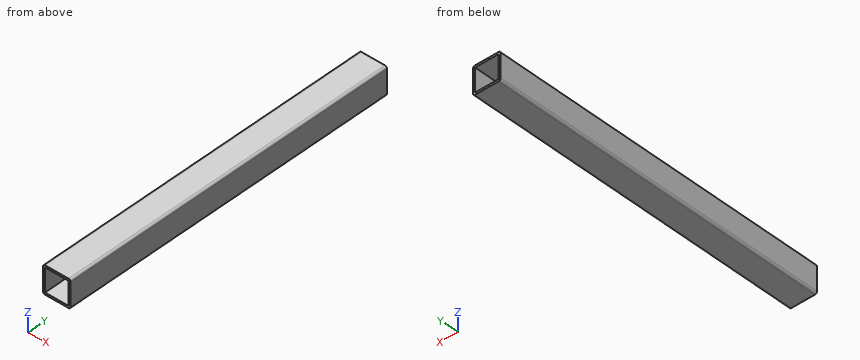
```python
from build123d import *

# Parameters (mm, degrees)
F0_W     = 34
F0_H     = 34
F1_DEPTH = 500


with BuildPart() as f1:
    # F0 (on Front) → F1 (new body)
    with BuildSketch(Plane.XZ):
        with BuildLine():
            ThreePointArc((19.779984, 17.078975), (18.901304, 19.200296), (16.779984, 20.078975))
            Line((16.779984, 20.078975), (-17.220016, 20.078975))
            ThreePointArc((-17.220016, 20.078975), (-19.341336, 19.200296), (-20.220016, 17.078975))
            Line((-20.220016, 17.078975), (-20.220016, -16.921025))
            ThreePointArc((-20.220016, -16.921025), (-19.341336, -19.042345), (-17.220016, -19.921025))
            Line((-17.220016, -19.921025), (16.779984, -19.921025))
            ThreePointArc((16.779984, -19.921025), (18.901304, -19.042345), (19.779984, -16.921025))
            Line((19.779984, -16.921025), (19.779984, 17.078975))
        make_face()
        with Locations((-0.220016, 0.078975)):
            Rectangle(F0_W, F0_H, mode=Mode.SUBTRACT)
    extrude(amount=F1_DEPTH)


solid = f1.part
```
Verification items for the finished model (mm, model axes). Round coordinates to 2 decimals unless told otherwise and drop trailing zeros. Order: outer loops, then holes, each group sorted by start corner. A loop starts at its lowest first (then second) coordinate and runs counter-clockwise, first axis right, second up. Notation, with made-up numbers: (54, 34.5) -> (72, 34.5) arc R11 ccw to (72, 53.5) -> close; hole circle Ø10 at (70.5, 10). An arc over 180 degrees is marked (long way). Put each result on its own line as item: value. Start each with the question number.
(1) Section check A-A (z = 6.5). Enter the section's corners in (x, y), then the cut area to 3 significant figures.
(2) Section check C-C (y = -262). Enter the section's corners in (x, z), then the cut area to 3 significant figures.
(3) Section check B-B (x = 0). Enter the section's corners in (y, z), then the cut area to 3 significant figures.
(4) Depth check by flat-ended pin: pin 1 Ø4 at (x, z) = (13, -2.5) entering from -Y. Enter the tip coordinate at first touch or a pass-through.
(5) Material ranges on line 1 along X through (y, z) = (-187, -1); line 2 along Z through (x, y) = (6, -162); line 3 along X through (y, z) = (-456.5, -17), recorded low to high.
Completed:
1. outline: (-20.22, -500) -> (-17.22, -500) -> (-17.22, 0) -> (-20.22, 0) -> close; (16.78, -500) -> (19.78, -500) -> (19.78, 0) -> (16.78, 0) -> close
1. area: 3,000 mm2
2. outline: (-20.22, -16.92) arc R3 ccw to (-17.22, -19.92) -> (16.78, -19.92) arc R3 ccw to (19.78, -16.92) -> (19.78, 17.08) arc R3 ccw to (16.78, 20.08) -> (-17.22, 20.08) arc R3 ccw to (-20.22, 17.08) -> close; hole (-17.22, -16.92) -> (16.78, -16.92) -> (16.78, 17.08) -> (-17.22, 17.08) -> close
2. area: 436 mm2
3. outline: (-500, -19.92) -> (0, -19.92) -> (0, -16.92) -> (-500, -16.92) -> close; (-500, 17.08) -> (0, 17.08) -> (0, 20.08) -> (-500, 20.08) -> close
3. area: 3,000 mm2
4. pin 1: passes through
5. line 1: x = -20.22 to -17.22, 16.78 to 19.78
5. line 2: z = -19.92 to -16.92, 17.08 to 20.08
5. line 3: x = -20.22 to 19.78
